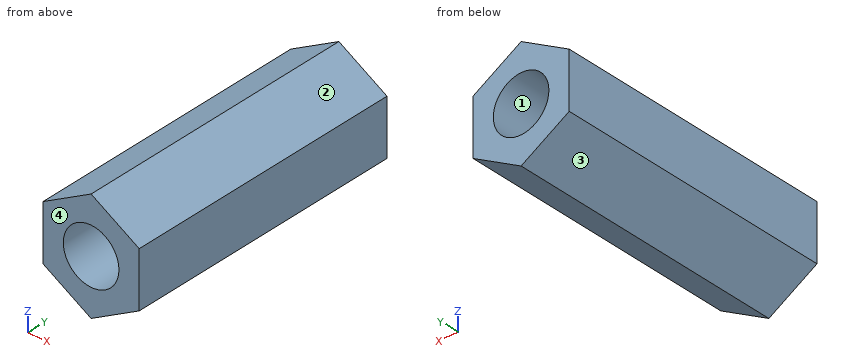
Autodesk Inventor part; units mm, degrees
ref_plane "YZ Plane" through (0, 0, 0) normal (1, 0, 0) x (0, 1, 0)
ref_plane "XZ Plane" through (0, 0, 0) normal (0, 1, 0) x (-1, 0, 0)
ref_plane "XY Plane" through (0, 0, 0) normal (0, 0, 1) x (1, 0, 0)
sketch "Sketch1" plane through (0, 0, 0) normal (0, 1, 0) x (-1, 0, 0)
  circle A0 centre (0, 0) radius 1.5
  line L0 (0, -3) -> (-2.5981, -1.5)
  line L1 (-2.5981, -1.5) -> (-2.5981, 1.5)
  line L2 (-2.5981, 1.5) -> (0, 3)
  line L3 (0, 3) -> (2.5981, 1.5)
  line L4 (2.5981, 1.5) -> (2.5981, -1.5)
  line L5 (2.5981, -1.5) -> (0, -3)
  dimension "d0" = 3
  dimension "d1" = 3
extrude "Extrusion1" add sketch "Sketch1" along normal blind 25
thread "Thread1"
sketch "Sketch2" plane through (0, 0, 0) normal (0, -1, 0) x (1, 0, 0)
  line L0 (-5.778, -4.3605) -> (5.778, -4.3605)
  line L1 (5.778, -4.3605) -> (5.778, 4.3605)
  line L2 (5.778, 4.3605) -> (-5.778, 4.3605)
  line L3 (-5.778, 4.3605) -> (-5.778, -4.3605)
  line L4 (-5.778, -4.3605) -> (5.778, 4.3605) construction
  line L5 (5.778, -4.3605) -> (-5.778, 4.3605) construction
  point P0 (0, 0)
extrude "Extrusion2" cut sketch "Sketch2" against normal blind 10
properties part number "dist25mm" material "Nylon 6/6"
For this review, take the finished solid that the model builds, in its own axes (mm). Face numbers are marked on the shaded views. Give positions to 0.01 mm unless a question says otherwise; leave off trailing zeros. Order: outer loops, then holes, each group sorted by start corner. A loop starts at its lowest first (then second) coordinate and runs counter-clockwise, first axis right, second up. Notation, with made-up numbers: (52, 45.25) - (61, 45.25) arc R8 cw to (61, 60.25) - close; hole circle Ø11 at (34, 55). An arc over 180 degrees is marked (long way). Answer as a JSON object with one key per item and string values. Group by question number.
Item 1: Wall thickness on line 1 along X through (y, z) = (19.5, 0); line 2 along X through (y, z) = (11.5, -0.85); line 3 along Z through (x, y) = (-0.75, 12.75): over which ranges is each line inside the solid? List them lowest first.
Item 2: Take a section at B-B on y = 12.5. Give the boundary of the cut face in (x, z), and give its area (3 significant figures).
Item 3: Clearance check with a flat-ended pin moving along its axis: pin 1 Ø2 at (x, y) = (2, 16) entering from +Z. State where the tip first meets the part, or that it passes through.
Item 4: Take a section at A-A on z = 0. Give the boundary of the cut face in (x, y).
Item 5: Draft analysis for pull direction X (two halves, no side actions). For the marked faces 1, 2, 3 and 4, state which applies: pulls with the +X half, pulls with the -X half, needs draft (parallel to the pull), parting line crosses it, or undercut.
Item 6: Take a section at D-D on x = -1.8. Give the boundary of the cut face in (y, z).
Item 7: Take a section at C-C on x = -0.25. Give the boundary of the cut face in (y, z), and give its area (3 significant figures).
Reported:
{
 "1": {"line 1": "-2.6 to -1.5, 1.5 to 2.6", "line 2": "-2.6 to -1.24, 1.24 to 2.6", "line 3": "-2.57 to -1.3, 1.3 to 2.57"},
 "2": {"outline": "(-2.6, -1.5) - (0, -3) - (2.6, -1.5) - (2.6, 1.5) - (0, 3) - (-2.6, 1.5) - close; hole circle Ø3 at (0, 0)", "area": "16.3 mm^2"},
 "3": {"pin 1": "z = 2.42"},
 "4": {"outline": "(-2.6, 10) - (-1.5, 10) - (-1.5, 25) - (-2.6, 25) - close; (1.5, 10) - (2.6, 10) - (2.6, 25) - (1.5, 25) - close"},
 "5": {"face 1": "undercut", "face 2": "pulls with the +X half", "face 3": "pulls with the -X half", "face 4": "needs draft"},
 "6": {"outline": "(10, -1.96) - (25, -1.96) - (25, 1.96) - (10, 1.96) - close"},
 "7": {"outline": "(10, -2.86) - (25, -2.86) - (25, -1.48) - (10, -1.48) - close; (10, 1.48) - (25, 1.48) - (25, 2.86) - (10, 2.86) - close", "area": "41.3 mm^2"}
}
